```python
from build123d import *

# Parameters (mm, degrees)
F0_R     = 3
F0_R_2   = 2.5
F1_DEPTH = 730.5
F2_R     = 2
F3_R     = 7


# Not quite as in the source:
# - a feature names something its author has since deleted; it is built from what else it names


with BuildPart() as f1:
    # F0 (on Top) → F1 (new body)
    with BuildSketch(Plane.XY):
        with BuildLine():
            Line((18.15, -15), (30, -15))
            Line((30, -15), (30, -3.15))
            Line((30, -3.15), (27.5, -3.15))
            Line((27.5, -3.15), (27.5, -5.15))
            Line((27.5, -5.15), (21.5477069044, -5.15))
            ThreePointArc((21.5477069044, -5.15), (19.5, 0), (21.5477069044, 5.15))
            Line((21.5477069044, 5.15), (27.5, 5.15))
            Line((27.5, 5.15), (27.5, 3.15))
            Line((27.5, 3.15), (30, 3.15))
            Line((30, 3.15), (30, 15))
            Line((30, 15), (18.15, 15))
            Line((18.15, 15), (18.15, 12.5))
            Line((18.15, 12.5), (20.15, 12.5))
            Line((20.15, 12.5), (20.15, 6.5477069044))
            ThreePointArc((20.15, 6.5477069044), (15, 4.5), (9.85, 6.5477069044))
            Line((9.85, 6.5477069044), (9.85, 12.5))
            Line((9.85, 12.5), (11.85, 12.5))
            Line((11.85, 12.5), (11.85, 15))
            Line((11.85, 15), (-11.85, 15))
            Line((-11.85, 15), (-11.85, 12.5))
            Line((-11.85, 12.5), (-9.85, 12.5))
            Line((-9.85, 12.5), (-9.85, 6.5477069044))
            ThreePointArc((-9.85, 6.5477069044), (-15, 4.5), (-20.15, 6.5477069044))
            Line((-20.15, 6.5477069044), (-20.15, 12.5))
            Line((-20.15, 12.5), (-18.15, 12.5))
            Line((-18.15, 12.5), (-18.15, 15))
            Line((-18.15, 15), (-30, 15))
            Line((-30, 15), (-30, 3.15))
            Line((-30, 3.15), (-27.5, 3.15))
            Line((-27.5, 3.15), (-27.5, 5.15))
            Line((-27.5, 5.15), (-21.5477069044, 5.15))
            ThreePointArc((-21.5477069044, 5.15), (-19.5, 0), (-21.5477069044, -5.15))
            Line((-21.5477069044, -5.15), (-27.5, -5.15))
            Line((-27.5, -5.15), (-27.5, -3.15))
            Line((-27.5, -3.15), (-30, -3.15))
            Line((-30, -3.15), (-30, -15))
            Line((-30, -15), (-18.15, -15))
            Line((-18.15, -15), (-18.15, -12.5))
            Line((-18.15, -12.5), (-20.15, -12.5))
            Line((-20.15, -12.5), (-20.15, -6.5477069044))
            ThreePointArc((-20.15, -6.5477069044), (-15, -4.5), (-9.85, -6.5477069044))
            Line((-9.85, -6.5477069044), (-9.85, -12.5))
            Line((-9.85, -12.5), (-11.85, -12.5))
            Line((-11.85, -12.5), (-11.85, -15))
            Line((-11.85, -15), (11.85, -15))
            Line((11.85, -15), (11.85, -12.5))
            Line((11.85, -12.5), (9.85, -12.5))
            Line((9.85, -12.5), (9.85, -6.5477069044))
            ThreePointArc((9.85, -6.5477069044), (15, -4.5), (20.15, -6.5477069044))
            Line((20.15, -6.5477069044), (20.15, -12.5))
            Line((20.15, -12.5), (18.15, -12.5))
            Line((18.15, -12.5), (18.15, -15))
        make_face()
        with Locations((-25, -10)):
            Circle(F0_R, mode=Mode.SUBTRACT)
        with Locations((25, -10)):
            Circle(F0_R, mode=Mode.SUBTRACT)
        with Locations((-15, 0)):
            Circle(F0_R_2, mode=Mode.SUBTRACT)
        with Locations((-25, 10)):
            Circle(F0_R, mode=Mode.SUBTRACT)
        Polygon((-7, 7), (-7, 12.5), (0, 12.5), (7, 12.5), (7, 7), (10, 0), (7, -7), (7, -12.5), (0, -12.5), (-7, -12.5), (-7, -7), (-10, 0), align=None, mode=Mode.SUBTRACT)
        with Locations((15, 0)):
            Circle(F0_R_2, mode=Mode.SUBTRACT)
        with Locations((25, 10)):
            Circle(F0_R, mode=Mode.SUBTRACT)
    extrude(amount=F1_DEPTH)

    # F2
    f2_edges = [f1.edges().sort_by_distance(p)[0] for p in [
        (-7, 12.5, 365.25),
        (7, 12.5, 365.25),
    ]]
    fillet(f2_edges, radius=F2_R)

    # F3
    f3_edges = [f1.edges().sort_by_distance(p)[0] for p in [
        (-7, 7, 365.25),
        (-10, 0, 365.25),
        (7, 7, 365.25),
        (10, 0, 365.25),
    ]]
    fillet(f3_edges, radius=F3_R)


solid = f1.part
```
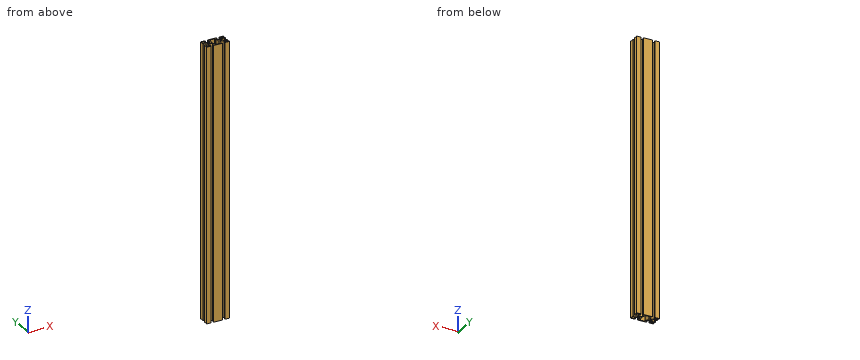
The listing builds one solid part. Answer for the finished solid, in the listing's coordinates (mm). Give positions to 0.01 mm unless a question says otherwise; leave off trailing zeros. Write each question's results on one line, items separated by ' | '.
Q1. The part is cut by section A-A, the plane z = 239. State how many separate pieces and enclosed holes the cut face has, and give its area (3 significant figures).
Checked values:
separate pieces: 1 | enclosed holes: 7 | area: 710 mm^2
Q2. Each of these flat-tipped pins is pushed along its axis until it touches: P1, Ø4, axis at x = -9, y = 8.5, coming from the -Z side; P2, Ø3, axis at x = -4.5, y = -4, coming from the -Z side. Where does it stop, or does it pass through?
Checked values:
P1: stops at z = 0 | P2: passes through
Q3. Straight lines are drawn through the part: probe 1 along X at (y, z) = (10.75, 553); probe 2 along X at (y, z) = (9.75, 357.5); probe 3 along Y at (x, z) = (25, 513). For each, find the intervals that lie inside material, in ascending order. Write a range as from..to.
Checked values:
probe 1: x = -30..-27.9, -22.1..-20.15, -9.85..-6.98, 6.98..9.85, 20.15..22.1, 27.9..30 | probe 2: x = -30..-27.99, -22.01..-20.15, -9.85..-7, 7..9.85, 20.15..22.01, 27.99..30 | probe 3: y = -15..-13, -7..-5.15, 5.15..7, 13..15
